Verification items for the finished model (mm, model axes). A direction names the side the tool comes from. Coordinates: 2 decimals unless noted, no trailing zeros. Loops run counter-clockwise (first coordinate to the right, second up) from the corner with the lowest first, then second, coordinate; pieces in that order, holes last. Notation, with made-up numbers: (-7, 66.5) -> (25, 66.5) arc R33 ccw to (25, 96.5) -> close; hole circle Ø5 at (-11, 34). An arc over 180 degrees is marked (long way). Use CSV: the item, a comma, the result in double quotes. Start each with the question number.
```python
from build123d import *

# Parameters (mm, degrees)
SKETCH1_R           = 1.5
SKETCH1_R_2         = 2
SKETCH1_W           = 3
SKETCH1_H           = 5
SKETCH1_H_2         = 7
BOSS_EXTRUDE1_DEPTH = 3


with BuildPart() as part:
    # Sketch1 → Boss-Extrude1 (new body)
    with BuildSketch(Plane(origin=(0, 0, 0), x_dir=(1, 0, 0), z_dir=(0, 1, 0))):
        with BuildLine():
            Line((11.699698215, 30.641238244), (11.699698215, 38.128019164))
            ThreePointArc((11.699698215, 38.128019164), (11.520568227, 38.955323461), (11.015265815, 39.634432749))
            ThreePointArc((11.015265815, 39.634432749), (-44.896357171, 60.611855364), (-100.807980157, 39.634432749))
            ThreePointArc((-100.807980157, 39.634432749), (-101.313282569, 38.955323461), (-101.492412558, 38.128019164))
            Line((-101.492412558, 38.128019164), (-101.492412558, 29.641238244))
            Line((-101.492412558, 29.641238244), (-98.492412558, 29.641238244))
            Line((-98.492412558, 29.641238244), (-98.492412558, 22.141238244))
            Line((-98.492412558, 22.141238244), (-95.492412558, 22.141238244))
            Line((-95.492412558, 22.141238244), (-95.492412558, 7.141238244))
            Line((-95.492412558, 7.141238244), (-98.492412558, 7.141238244))
            Line((-98.492412558, 7.141238244), (-98.492412558, -22.858761756))
            Line((-98.492412558, -22.858761756), (-95.492412558, -22.858761756))
            Line((-95.492412558, -22.858761756), (-95.492412558, -37.858761756))
            Line((-95.492412558, -37.858761756), (-98.492412558, -37.858761756))
            Line((-98.492412558, -37.858761756), (-98.492412558, -40.358761756))
            Line((-98.492412558, -40.358761756), (-100.492412558, -40.358761756))
            ThreePointArc((-100.492412558, -40.358761756), (-101.199519339, -40.651654975), (-101.492412558, -41.358761756))
            Line((-101.492412558, -41.358761756), (-101.492412558, -46.358761756))
            ThreePointArc((-101.492412558, -46.358761756), (-101.785305776, -47.065868537), (-102.492412558, -47.358761756))
            Line((-102.492412558, -47.358761756), (-124.051068216, -47.358761756))
            ThreePointArc((-124.051068216, -47.358761756), (-125.664047329, -48.176265083), (-125.958410651, -49.960463374))
            ThreePointArc((-125.958410651, -49.960463374), (-44.896357171, -109.388144636), (36.165696309, -49.960463373))
            ThreePointArc((36.165696309, -49.960463373), (35.871332987, -48.176265083), (34.258353874, -47.358761756))
            Line((34.258353874, -47.358761756), (12.699698215, -47.358761756))
            ThreePointArc((12.699698215, -47.358761756), (11.992591434, -47.065868537), (11.699698215, -46.358761756))
            Line((11.699698215, -46.358761756), (11.699698215, -41.358761756))
            ThreePointArc((11.699698215, -41.358761756), (11.406804997, -40.651654975), (10.699698215, -40.358761756))
            Line((10.699698215, -40.358761756), (8.699698215, -40.358761756))
            Line((8.699698215, -40.358761756), (8.699698215, -37.858761756))
            Line((8.699698215, -37.858761756), (5.699698215, -37.858761756))
            Line((5.699698215, -37.858761756), (5.699698215, -22.858761756))
            Line((5.699698215, -22.858761756), (8.699698215, -22.858761756))
            Line((8.699698215, -22.858761756), (8.699698215, 7.141238244))
            Line((8.699698215, 7.141238244), (5.699698215, 7.141238244))
            Line((5.699698215, 7.141238244), (5.699698215, 22.141238244))
            Line((5.699698215, 22.141238244), (8.699698215, 22.141238244))
            Line((8.699698215, 22.141238244), (8.699698215, 29.641238244))
            Line((8.699698215, 29.641238244), (10.699698215, 29.641238244))
            ThreePointArc((10.699698215, 29.641238244), (11.406804996, 29.934131463), (11.699698215, 30.641238244))
        make_face()
        with Locations(Location((2.199698215, 30.187503495, 0), (0, 0, 270))):
            Circle(SKETCH1_R, mode=Mode.SUBTRACT)
        with Locations(Location((2.199698215, -45.858761756, 0), (0, 0, 270))):
            Circle(SKETCH1_R, mode=Mode.SUBTRACT)
        with Locations(Location((-91.992412558, -45.858761756, 0), (0, 0, 270))):
            Circle(SKETCH1_R, mode=Mode.SUBTRACT)
        with Locations(Location((-91.992412558, 30.187503495, 0), (0, 0, 270))):
            Circle(SKETCH1_R, mode=Mode.SUBTRACT)
        with Locations(Location((-24.942412558, -87.858761756, 0), (0, 0, 270))):
            Circle(SKETCH1_R_2, mode=Mode.SUBTRACT)
        with Locations(Location((-64.542412558, -87.858761756, 0), (0, 0, 270))):
            Circle(SKETCH1_R_2, mode=Mode.SUBTRACT)
        with Locations((-96.992412558, -44.858761756)):
            Rectangle(SKETCH1_W, SKETCH1_H, mode=Mode.SUBTRACT)
        with Locations((7.199698215, 35.141238244)):
            Rectangle(SKETCH1_W, SKETCH1_H_2, mode=Mode.SUBTRACT)
        with Locations((7.199698215, -44.858761756)):
            Rectangle(SKETCH1_W, SKETCH1_H, mode=Mode.SUBTRACT)
        with BuildLine():
            Line((-75.492412558, 16.141238244), (-73.492412558, 16.141238244))
            ThreePointArc((-73.492412558, 16.141238244), (-68.542665089, 14.090985712), (-66.492412558, 9.141238244))
            Line((-66.492412558, 9.141238244), (-66.492412558, -10.829459129))
            ThreePointArc((-66.492412558, -10.829459129), (-68.542665089, -15.779206597), (-73.492412558, -17.829459129))
            Line((-73.492412558, -17.829459129), (-75.492412558, -17.829459129))
            ThreePointArc((-75.492412558, -17.829459129), (-80.442160026, -15.779206597), (-82.492412558, -10.829459129))
            Line((-82.492412558, -10.829459129), (-82.492412558, 9.141238244))
            ThreePointArc((-82.492412558, 9.141238244), (-80.442160026, 14.090985712), (-75.492412558, 16.141238244))
        make_face(mode=Mode.SUBTRACT)
        with Locations((-96.992412558, 35.141238244)):
            Rectangle(SKETCH1_W, SKETCH1_H_2, mode=Mode.SUBTRACT)
        with BuildLine():
            Line((-29.896357171, 23.611855364), (-29.896357171, 8.611855364))
            ThreePointArc((-29.896357171, 8.611855364), (-30.775036828, 6.49053502), (-32.896357171, 5.611855364))
            Line((-32.896357171, 5.611855364), (-36.896357171, 5.611855364))
            ThreePointArc((-36.896357171, 5.611855364), (-39.017677515, 6.49053502), (-39.896357171, 8.611855364))
            Line((-39.896357171, 8.611855364), (-39.896357171, 23.611855364))
            ThreePointArc((-39.896357171, 23.611855364), (-39.017677515, 25.733175707), (-36.896357171, 26.611855364))
            Line((-36.896357171, 26.611855364), (-32.896357171, 26.611855364))
            ThreePointArc((-32.896357171, 26.611855364), (-30.775036828, 25.733175707), (-29.896357171, 23.611855364))
        make_face(mode=Mode.SUBTRACT)
        with BuildLine():
            Line((-56.896357171, 5.611855364), (-52.896357171, 5.611855364))
            ThreePointArc((-52.896357171, 5.611855364), (-50.775036828, 6.49053502), (-49.896357171, 8.611855364))
            Line((-49.896357171, 8.611855364), (-49.896357171, 23.611855364))
            ThreePointArc((-49.896357171, 23.611855364), (-50.775036828, 25.733175707), (-52.896357171, 26.611855364))
            Line((-52.896357171, 26.611855364), (-56.896357171, 26.611855364))
            ThreePointArc((-56.896357171, 26.611855364), (-59.017677515, 25.733175707), (-59.896357171, 23.611855364))
            Line((-59.896357171, 23.611855364), (-59.896357171, 8.611855364))
            ThreePointArc((-59.896357171, 8.611855364), (-59.017677515, 6.49053502), (-56.896357171, 5.611855364))
        make_face(mode=Mode.SUBTRACT)
        with BuildLine():
            Line((-7.300301785, 9.141238244), (-7.300301785, -10.829459129))
            ThreePointArc((-7.300301785, -10.829459129), (-9.350554316, -15.779206597), (-14.300301785, -17.829459129))
            Line((-14.300301785, -17.829459129), (-16.300301785, -17.829459129))
            ThreePointArc((-16.300301785, -17.829459129), (-21.250049253, -15.779206597), (-23.300301785, -10.829459129))
            Line((-23.300301785, -10.829459129), (-23.300301785, 9.141238244))
            ThreePointArc((-23.300301785, 9.141238244), (-21.250049253, 14.090985712), (-16.300301785, 16.141238244))
            Line((-16.300301785, 16.141238244), (-14.300301785, 16.141238244))
            ThreePointArc((-14.300301785, 16.141238244), (-9.350554316, 14.090985712), (-7.300301785, 9.141238244))
        make_face(mode=Mode.SUBTRACT)
    extrude(amount=BOSS_EXTRUDE1_DEPTH)


solid = part.part
```
1. Cross-section at D-D, the plane y = 2.55. State how many separate pieces and enclosed holes the cut face has, plus the area to 3 significant figures.
2. Release check for a two-part mould opening along Z. For faces 3 (the cylindrical face through (-68.489, 1.479, 15.724)), 4 (the cylindrical face through (-46.402, 1.479, 109.375)), 5 (the cylindrical face through (-44.042, 1.479, -60.608)) record: released by +Z, released by -Z, zero draft, split by the parting line, or undercut.
3. Depth check by flat-ended pin: pin 1 (1.6 mm diameter, centred on x = -15.5, y = 2, fed in from -Z); pin 2 (0.9 mm diameter, centred on y = 1, z = -16, fed in from +X); pin 3 (1.5 mm diameter, centred on y = 2, z = 30.5, fed in from -X); pin 4 (2 mm diameter, centred on x = -89, z = 40.5, fed in from -Y). Enter the tip coordinate at first touch or a pass-through.
4. Cross-section at B-B, the plane x = -78.5. Record the boundary of the cut face in (y, z), plus the area to 3 significant figures.
5. Scan lines: line 1 (X direction, y = 1.05, z = 3.5); line 2 (X direction, y = 1, z = -8.5); line 3 (Z direction, x = 1, y = 0.75). Record each from-to range of solid material in increasing order.
6. Cross-section at A-A, the plane z = 2.5. Record the boundary of the cut face in (x, y), plus the area to 3 significant figures.
7. Set-up check for faces 1 (the flat face through (-46, 0, 23)), 2 (the cylindrical face through (-21.3, 1.48, -14.04)): record each of +Z, -Z, +X, -X, +Y, -Y from which the full face is reachable in a straight line by a thin tool's end or side.
8. Cross-section at C-C, the plane x = -20.5. Record the boundary of the cut face in (y, z).
Solution:
1,separate pieces,"1"
1,enclosed holes,"14"
1,area,"16,800 mm2"
2,face 3,"undercut"
2,face 4,"released by +Z"
2,face 5,"released by -Z"
3,pin 1,"stops at z = -55.66"
3,pin 2,"stops at x = 5.7"
3,pin 3,"stops at x = -95.49"
3,pin 4,"stops at y = 0"
4,outline,"(0, -53.69) -> (3, -53.69) -> (3, -15.46) -> (0, -15.46) -> close; (0, 17.15) -> (3, 17.15) -> (3, 102.46) -> (0, 102.46) -> close"
4,area,"371 mm2"
5,line 1,"x = -98.49 to -82.49, -66.49 to -23.3, -7.3 to 8.7"
5,line 2,"x = -95.49 to -82.49, -66.49 to -59.89, -49.9 to -39.89, -29.9 to -23.3, -7.3 to 5.7"
5,line 3,"z = -47.16 to -31.09, -29.29 to 44.96, 46.76 to 95.93"
6,outline,"(-98.49, 0) -> (-82.49, 0) -> (-82.49, 3) -> (-98.49, 3) -> close; (-66.49, 0) -> (-23.3, 0) -> (-23.3, 3) -> (-66.49, 3) -> close; (-7.3, 0) -> (8.7, 0) -> (8.7, 3) -> (-7.3, 3) -> close"
6,area,"226 mm2"
7,face 1,"+Z, -Z, +X, -X, -Y"
7,face 2,"+Y, -Y"
8,outline,"(0, -57.04) -> (3, -57.04) -> (3, -14.74) -> (0, -14.74) -> close; (0, 16.43) -> (3, 16.43) -> (3, 105.81) -> (0, 105.81) -> close"
